Build history of the part. All positions in model axes, mm. Face numbers are marked on the shaded views. A direction names the side the tool comes from. Round coordinates to 2 decimals unless told otherwise and drop trailing zeros. Write each loop counter-clockwise with the first axis right and the second up, starting at its lowest first coordinate (ties: lowest second). Pieces come first, ordered by that corner, then holes.
1) Saw through at A-A (x = 22). Write the cut outline in (y, z), plus the area to 3 significant figures.
2) Which spindle directions (+Z, -Z, +X, -X, +Y, -Y) get a long thin tool onto all of the face, cutting with end or side? Do the marked faces 4 and 5. Say none if no direction does.
3) Saw through at B-B (y = 57). State how many separate pieces and enclosed holes the cut face has, plus the area to 3 significant figures.
4) Wall check: probe 1 along Y at (x, z) = (-16, 0); probe 2 along Y at (x, z) = (-7.5, 0); probe 3 along Z at (x, y) = (-21, 24). Give the ranges that are in metal, low to high.
5) Flat gauge pins, fed straight in: pin 1 (6 mm diameter, centred on x = -13, y = -17, fed in from +Z); pin 2 (1 mm diameter, centred on x = 20.5, y = 6.5, fed in from -Z); pin 3 (5 mm diameter, centred on x = 3.5, z = 0.5, fed in from -Y). Where does each tip first touch, or does it go through?
6) Pull direction Y, two halves, no side cores. Call the marked faces 1, 2 and 3: +Y half, -Y half, draft (parallel to the pull), parting line (faces both ways), or undercut.
from build123d import *

# Parameters (mm, degrees)
SKETCH_1_R             = 65.25
EXTRUDE_1_DEPTH        = 31.5
PATTERN_LINEAR_1_COUNT = 4
PATTERN_LINEAR_1_PITCH = 15


with BuildPart() as part:
    # 草图1 → 凸台-拉伸1 (new, symmetric)
    with BuildSketch(Plane(origin=(0, 0, 0), x_dir=(0, 0, -1), z_dir=(1, 0, 0))):
        Circle(SKETCH_1_R)
        with BuildLine():
            Line((-5, 14.142135624), (-5, 25))
            Line((-5, 25), (5, 25))
            Line((5, 25), (5, 14.142135624))
            ThreePointArc((5, 14.142135624), (0, -15), (-5, 14.142135624))
        make_face(mode=Mode.SUBTRACT)
    extrude(amount=EXTRUDE_1_DEPTH, both=True)

    # 草图2 → 切除-旋转1 (revolve, cut)
    with BuildSketch(Plane.XY, mode=Mode.PRIVATE) as cut_revolve_1_sk:
        Polygon((-28.840759374, 65.25), (-16.159240626, 65.25), (-19.659856929, 53.8), (-25.340143071, 53.8), align=None)
    cut_revolve_1 = revolve(cut_revolve_1_sk.sketch.rotate(Axis((0, 0, 0), (1, 0, 0)), 90), axis=Axis((0, 0, 0), (1, 0, 0)), mode=Mode.SUBTRACT)

    # 阵列(线性)1: 切除-旋转1 ×4
    with Locations(*[(i * PATTERN_LINEAR_1_PITCH, 0, 0) for i in range(1, PATTERN_LINEAR_1_COUNT)]):
        add(cut_revolve_1, mode=Mode.SUBTRACT)


solid = part.part
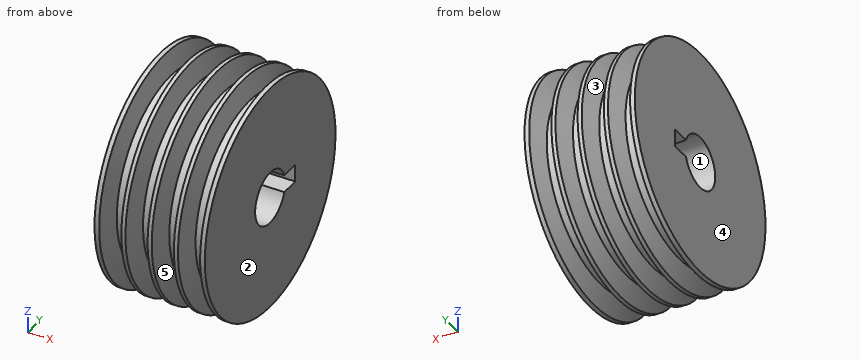
Evaluation:
1. outline: circle Ø107.6 at (0, 0); hole (14.14, -5) - (25, -5) - (25, 5) - (14.14, 5) arc R15 ccw (long way) to start
1. area: 8,280 mm2
2. face 4: +Z, -Z, -X, +Y, -Y
2. face 5: none
3. separate pieces: 5
3. enclosed holes: 0
3. area: 1,620 mm2
4. probe 1: y = -65.25 to -15, 25 to 65.25
4. probe 2: y = -53.8 to -15, 25 to 53.8
4. probe 3: z = -48.15 to -5, 5 to 48.15
5. pin 1: stops at z = 63.7
5. pin 2: stops at z = -53.46
5. pin 3: stops at y = -65.25
6. face 1: undercut
6. face 2: draft
6. face 3: parting line
